Design review of the part shown in the three views and the two pictorial views. Dimensions are in mm from the part's minimum x, y and z. A direction names the side the tool comes from. Coordinates: 2 decimals unless noted, no trailing zeros. Loops run counter-clockwise (first coordinate to the right, second up) from the corner with the lowest first, then second, coordinate; pieces in that order, holes last. Notation, with made-up numbers: (-26.5, -31) -> (31.5, -31) arc R22 cw to (31.5, -1) -> close; hole circle Ø3 at (73.5, 35.25). An arc over 180 degrees is marked (long way). Use a Markdown table: item, result. Add a question column.
Q1. For the marked faces 1, 2, 3 and 4, list the 3-axis set-ups (+Z, -Z, +X, -X, +Y, -Y) from which the entire face can be reached by the end or side of a thin tool; tool diameter is ignored.
Q2. Take a section at D-D on y = 111. Write out the cut boundary in (x, z).
Q3. Clearance check with flat-ended pins moving along their axes: pin 1 Ø19 at (x, z) = (109, 10) entering from +Y; pin 2 Ø4 at (x, y) = (22, 117.5) entering from -Z; pin 3 Ø2 at (x, y) = (108.5, 41.5) entering from -Z. State where each tip first meets the part, or that it passes through.
Q4. For probe 1 along Y at (x, z) = (150, 69); probe 2 along Z at (x, y) = (76, 80), list the stretches that pass through material, from the lowest coordinate up.
Q5. Take a section at B-B on y = 59.5. Write out the cut boundary in (x, z), plus the area to 4 significant figures.
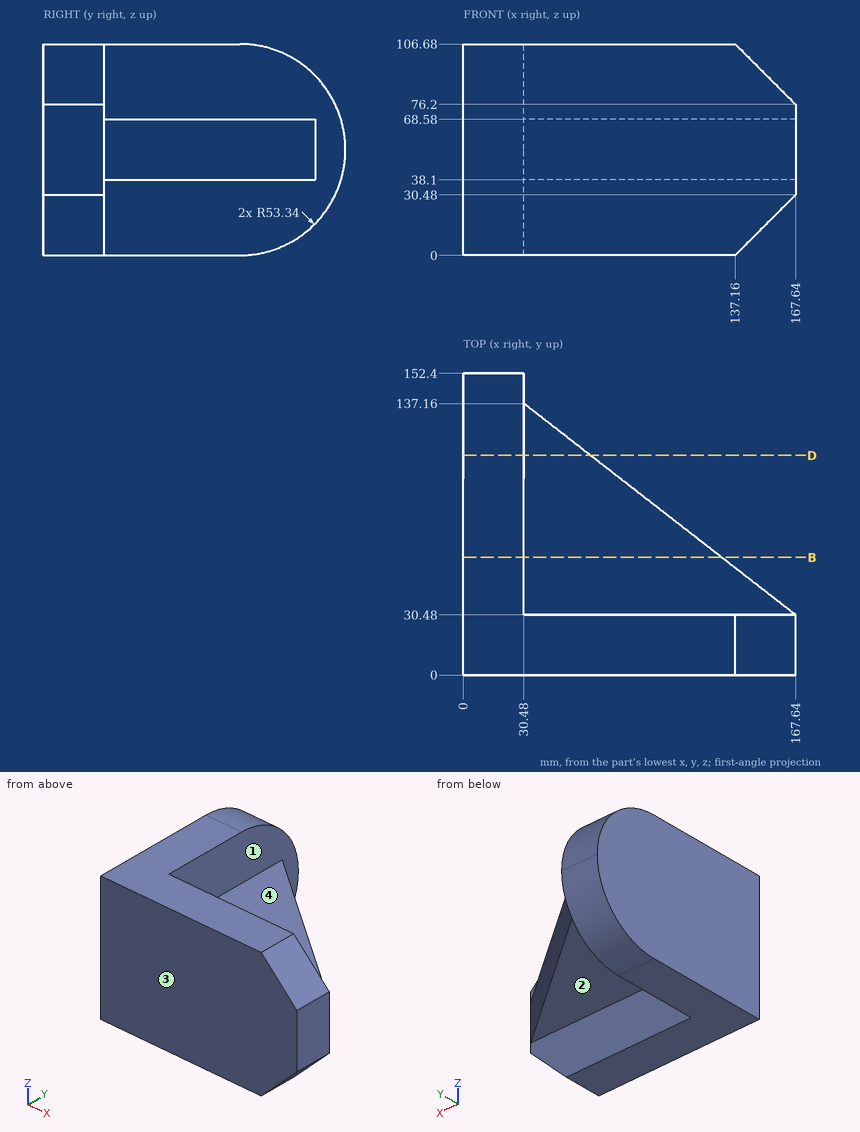
Answer list:
| question | item | result |
|---|---|---|
| 1 | face 1 | +X, +Y |
| 1 | face 2 | -Z, +X, +Y |
| 1 | face 3 | +Z, -Z, +X, -X, -Y |
| 1 | face 4 | +Z, +X, +Y |
| 2 | outline | (0, 1.35) -> (30.48, 1.35) -> (30.48, 38.1) -> (64.11, 38.1) -> (64.11, 68.58) -> (30.48, 68.58) -> (30.48, 105.33) -> (0, 105.33) -> close |
| 3 | pin 1 | y = 30.48 |
| 3 | pin 2 | z = 2.6 |
| 3 | pin 3 | z = 38.1 |
| 4 | probe 1 | 0 to 30.48 |
| 4 | probe 2 | 38.1 to 68.58 |
| 5 | outline | (0, 0) -> (30.48, 0) -> (30.48, 38.1) -> (130.33, 38.1) -> (130.33, 68.58) -> (30.48, 68.58) -> (30.48, 106.68) -> (0, 106.68) -> close |
| 5 | area | 6,295 mm² |
